CAD build for the part. Positions are in the model's coordinates, mm. Face numbers are marked on the shaded views. A direction names the side the tool comes from. Give positions to 0.01 mm unless a question says otherwise; leave off trailing zeros. Order: outer loops, then holes, each group sorted by start corner. A loop starts at its lowest first (then second) coordinate and runs counter-clockwise, first axis right, second up. Notation, with made-up numbers: M 0.25,45.25 L 50.25,45.25 A23 ccw 50.25,81.25 Z; hole C -15.75,30.5 d3. An arc over 180 degrees is marked long. Put each result on its own line as item: value. Start each with the question number.
1) Cut at B-B (z = -0.5). Write the cut outline in (x, y).
2) Cut at A-A (y = 9.4). Write the cut outline in (x, z).
3) Cut at C-C (x = 19.5). Write the cut outline in (y, z).
4) Drill centre lines: line 1 (Z direction, x = 20.5, y = 8.65); line 2 (X direction, y = 6.55, z = -15). Where is each one in solid material? Low to high. Write a range as [from, to].
5) Tool access for the marked faces 1 and 2: list every direction of +Z, -Z, +X, -X, +Y, -Y with a clear straight run to the whole face (end or side of a thin tool).
6) Pin check, flat tips, straight feed: pin 1 (1 mm diameter, centred on y = 6.5, z = -7.5, fed in from -X); pin 2 (1.5 mm diameter, centred on x = 19.5, y = 7, fed in from -Z); pin 3 (2.5 mm diameter, centred on y = 6.5, z = -1.5, fed in from -X). Stop position of each tip, or through.
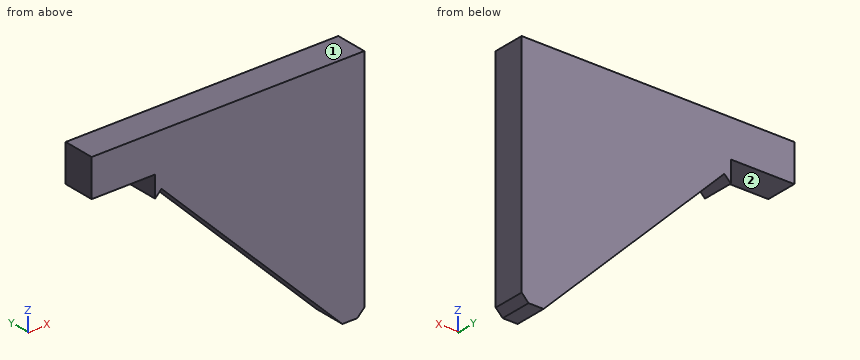
```python
from build123d import *

# Parameters (mm, degrees)
BOX010_W               = 5
BOX010_H               = 85
BOX010_DEPTH           = 42
BOX010_PLACEMENT_ANGLE = 315
BOX007_W               = 7
BOX007_H               = 5
BOX007_DEPTH           = 36.85
BOX_W                  = 50
BOX_H                  = 5
BOX_DEPTH              = 5.85
BOX004_W               = 24
BOX004_H               = 85
BOX004_DEPTH           = 42
BOX004_PLACEMENT_ANGLE = 315
BOX002_W               = 40
BOX002_H               = 5
BOX002_DEPTH           = 30.85


with BuildPart() as cube010:
    # Box010 → Box010 (new body)
    with BuildSketch(Plane.XY):
        with Locations((2.5, 42.5)):
            Rectangle(BOX010_W, BOX010_H)
    extrude(amount=BOX010_DEPTH)


with BuildPart() as cube010_1:
    # Box010 placement: moved
    add(cube010.part.moved(Location((82.4, 5, -62))).rotate(Axis((82.4, 5, -62), (0, 1, 0)), BOX010_PLACEMENT_ANGLE))


with BuildPart() as cube007:
    # Box007 → Box007 (new body)
    with BuildSketch(Plane(origin=(55.25, 5, -31), x_dir=(1, 0, 0), z_dir=(0, 0, 1))):
        with Locations((3.5, 2.5)):
            Rectangle(BOX007_W, BOX007_H)
    extrude(amount=BOX007_DEPTH)


with BuildPart() as cube:
    # Box → Box (new body)
    with BuildSketch(Plane(origin=(12.25, 5, 0), x_dir=(1, 0, 0), z_dir=(0, 0, 1))):
        with Locations((25, 2.5)):
            Rectangle(BOX_W, BOX_H)
    extrude(amount=BOX_DEPTH)


with BuildPart() as cube004:
    # Box004 → Box004 (new body)
    with BuildSketch(Plane.XY):
        with Locations((12, 42.5)):
            Rectangle(BOX004_W, BOX004_H)
    extrude(amount=BOX004_DEPTH)


with BuildPart() as cube004_1:
    # Box004 placement: moved
    add(cube004.part.moved(Location((36, 5, -49))).rotate(Axis((36, 5, -49), (0, 1, 0)), BOX004_PLACEMENT_ANGLE))


with BuildPart() as cut005:
    # Box002 → Box002 (new body)
    with BuildSketch(Plane(origin=(22.25, 5, -30.85), x_dir=(1, 0, 0), z_dir=(0, 0, 1))):
        with Locations((20, 2.5)):
            Rectangle(BOX002_W, BOX002_H)
    extrude(amount=BOX002_DEPTH)

    # Cut: cut Cube004
    add(cube004_1.part, mode=Mode.SUBTRACT)

    # Fusion: union Cube
    add(cube.part)

    # Cut002: cut Cube007
    add(cube007.part, mode=Mode.SUBTRACT)

    # Cut005: cut Cube010
    add(cube010_1.part, mode=Mode.SUBTRACT)


solid = cut005.part
```
Solution:
1. outline: M 22.25,5 L 55.25,5 L 55.25,10 L 22.25,10 Z
2. outline: M 12.25,0 L 22.25,0 L 22.25,-3.35 L 23.27,-2.33 L 51.79,-30.85 L 54.15,-30.85 L 55.25,-29.75 L 55.25,5.85 L 12.25,5.85 Z
3. outline: M 5,0 L 10,0 L 10,5.85 L 5,5.85 Z
4. line 1: [0, 5.85]
4. line 2: [35.94, 55.25]
5. face 1: +Z, +X, -X, +Y, -Y
5. face 2: -Z, -X, +Y, -Y
6. pin 1: x = 27.94
6. pin 2: z = 0
6. pin 3: x = 22.25
